The drawing under review shows one solid part. Ordinate dimensions are in mm from its lowest x, y, z. A direction names the side the tool comes from. Round coordinates to 2 decimals unless told otherwise and drop trailing zeros. Write each loop counter-clockwise with the first axis right and the second up, starting at its lowest first coordinate (ties: lowest second). Pieces come first, ordered by that corner, then holes. Notation, with made-up numbers: (89, 42.5) -> (94, 42.5) arc R22 ccw to (94, 66.5) -> close; hole circle Ø5 at (19.5, 8.25). An arc over 180 degrees is marked (long way). Write item = value, one per line. Start each with the question number.
Item 1: Add section D-D, the plane z = 12.9. State the section outline as (x, y) points, then the cut area to 3 significant figures.
Item 2: Mouldability with a two-part tool opening along X and no side actions: class the marked faces 6, 7 and 8 as released by +X, released by -X, zero draft, split by the parting line, or undercut.
Item 3: To check wall thickness, follow L1, parallel to Z at x = 48.5, y = 5.75; L2, parallel to Z at x = 27, y = 3.75; L3, parallel to X at y = 9.5, z = 31.5. State the ranges of each line that lie inside material, in increasing order.
Item 4: Add section C-C, the plane x = 54. State the section outline as (y, z) points.
Item 5: For pin 1 Ø6 at (x, z) = (41, 32.5) entering from +Y, flat-tipped, find the tip position at first contact; note if it passes through.
Item 6: Add section B-B, the plane x = 26.5. State the section outline as (y, z) points.
Item 7: Machinability: for the marked faces 1, 2, 3, 4 and 5, which of the approach directions +Z, -Z, +X, -X, +Y, -Y give a long, thin tool a straight path to every point of the face, cutting with its end or side? Answer none if there is none.
Item 8: Add section A-A, the plane z = 57.1. State the section outline as (x, y) points, then the cut area to 3 significant figures.
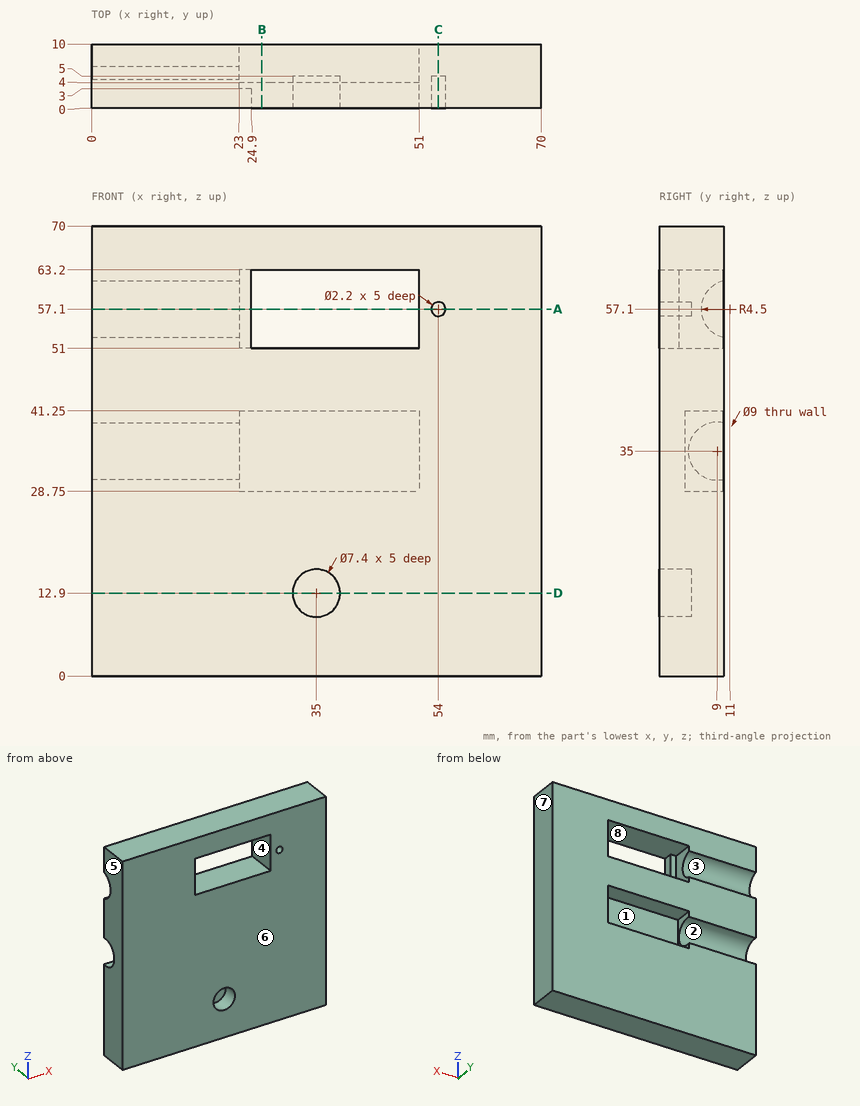
Result set:
q1.outline = (0, 0) -> (31.3, 0) -> (31.3, 5) -> (38.7, 5) -> (38.7, 0) -> (70, 0) -> (70, 10) -> (0, 10) -> close
q1.area = 663 mm²
q2.face_6 = zero draft
q2.face_7 = released by +X
q2.face_8 = undercut
q3.L1 = 0 to 28.75, 41.25 to 51, 63.2 to 70
q3.L2 = 0 to 51, 63.2 to 70
q3.L3 = 51 to 70
q4.outline = (0, 0) -> (10, 0) -> (10, 70) -> (0, 70) -> (0, 58.2) -> (5, 58.2) -> (5, 56) -> (0, 56) -> close
q5.pin_1 = 4
q6.outline = (0, 0) -> (10, 0) -> (10, 28.75) -> (4, 28.75) -> (4, 41.25) -> (10, 41.25) -> (10, 51) -> (0, 51) -> close; (0, 63.2) -> (10, 63.2) -> (10, 70) -> (0, 70) -> close
q7.face_1 = +Y
q7.face_2 = -X
q7.face_3 = -X, +Y
q7.face_4 = +Y, -Y
q7.face_5 = +Z, -Z, -X, +Y, -Y
q8.outline = (0, 0) -> (24.9, 0) -> (24.9, 3) -> (23, 3) -> (23, 6.5) -> (0, 6.5) -> close; (51, 0) -> (52.9, 0) -> (52.9, 5) -> (55.1, 5) -> (55.1, 0) -> (70, 0) -> (70, 10) -> (51, 10) -> close
q8.area = 334 mm²
